Source: CAD feature listing. Evaluate the final solid. Frame: model axes, mm. A direction names the side the tool comes from. Round coordinates to 2 decimals unless told otherwise and drop trailing zeros. Order: outer loops, then holes, each group sorted by start corner. A loop starts at its lowest first (then second) coordinate and runs counter-clockwise, first axis right, second up. Notation, with made-up numbers: (54.25, 87) -> (68.25, 87) arc R27 ccw to (68.25, 104) -> close; hole circle Ø8 at (48.25, -36). An arc over 180 degrees is marked (long way). One line per item, written item: value. Start each with the question number.
1) Section A-A (y = 0). Return the cut outline in (x, z), and give its area (3 significant figures).
2) Pin query (flat end, axial travel): P1, Ø4, axis at x = 18, z = 536.5, coming from the -Y side; P2, Ø16, axis at y = 0, z = 325, coming from the -X side; P3, Ø15.5, axis at x = -24.5, y = 3, coming from the -Z side; P4, Ø6, axis at y = 0.5, z = 429.5, coming from the -X side. Return the tip coordinate at first contact, or that it passes through.
3) Section D-D (z = 522.5). Return the cut outline in (x, y), and give its area (3 significant figures).
4) Section B-B (x = 0). Return the cut outline in (y, z).
5) Ray query, L1, parallel to Z at x = -4, y = 0; L2, parallel to Z at x = -11, y = -9; L3, parallel to X at y = -5, z = 335. Return the intervals inside material, ascending.
6) Reachability of faces 5 (the face through (-4.336, -19.524, 524.865)), 6 (the face through (15, 0, 197)), 7 (the face through (0, -25, 197)), 8 (the face through (0, 25, 197)) from +Z, -Z, +X, -X, +Y, -Y: full face, straight path, thin tool, end or side. Return the list, or none.
7) Section C-C (z = 125). Return the cut outline in (x, y).
8) Mould query, pull axis Z, two halves, no side actions, for faces 1 (the face through (-22, 1, 400)), 2 (the face through (0.21, -1.302, 334.915)), 3 (the face through (-15, 0, 197)), 4 (the face through (0.21, -1.302, 34.915)). Classes: pulls with the +Z half, pulls with the -Z half, needs draft (parallel to the pull), parting line crosses it, or undercut.
```python
from build123d import *

# Parameters (mm, degrees)
ESQUISSE1_W             = 30
ESQUISSE1_H             = 50
BOSS_EXTRU_1_DEPTH      = 400
ESQUISSE2_R             = 29.154759474
BOSS_EXTRU_2_DEPTH      = 221
ESQUISSE3_R             = 20
ENL_V_MAT_EXTRU_1_DEPTH = 195
ENL_V_MAT_EXTRU_2_REACH = 625.25
ESQUISSE4_R             = 10


with BuildPart() as part:
    # Esquisse1 → Boss.-Extru.1 (new body)
    with BuildSketch(Plane.XY):
        Rectangle(ESQUISSE1_W, ESQUISSE1_H)
    extrude(amount=BOSS_EXTRU_1_DEPTH)

    # Esquisse2 → Boss.-Extru.2 (add)
    with BuildSketch(Plane.XY.offset(400)):
        with Locations(Location((0, 0, 0), (0, 0, 120.963756532))):
            Circle(ESQUISSE2_R)
    extrude(amount=BOSS_EXTRU_2_DEPTH)

    # Esquisse3 → Enlèv. mat.-Extru.1 (cut)
    with BuildSketch(Plane.XY.offset(621)):
        Circle(ESQUISSE3_R)
    extrude(amount=-ENL_V_MAT_EXTRU_1_DEPTH, mode=Mode.SUBTRACT)

    # Esquisse4 → Enlèv. mat.-Extru.2 (cut, up to next)
    with BuildSketch(Plane(origin=(15, 0, 0), x_dir=(0, 0, -1), z_dir=(1, 0, 0)), mode=Mode.PRIVATE) as enl_v_mat_extru_2_sk1:
        with Locations(Location((-25, 0, 0), (0, 0, 90))):
            Circle(ESQUISSE4_R)
    enl_v_mat_extru_2_tool1 = extrude(enl_v_mat_extru_2_sk1.sketch, amount=-ENL_V_MAT_EXTRU_2_REACH, mode=Mode.PRIVATE) & part.part
    # Esquisse4 → Enlèv. mat.-Extru.2 (cut, up to next)
    with BuildSketch(Plane(origin=(15, 0, 0), x_dir=(0, 0, -1), z_dir=(1, 0, 0)), mode=Mode.PRIVATE) as enl_v_mat_extru_2_sk2:
        with Locations(Location((-125, 0, 0), (0, 0, 90))):
            Circle(ESQUISSE4_R)
    enl_v_mat_extru_2_tool2 = extrude(enl_v_mat_extru_2_sk2.sketch, amount=-ENL_V_MAT_EXTRU_2_REACH, mode=Mode.PRIVATE) & part.part
    # Esquisse4 → Enlèv. mat.-Extru.2 (cut, up to next)
    with BuildSketch(Plane(origin=(15, 0, 0), x_dir=(0, 0, -1), z_dir=(1, 0, 0)), mode=Mode.PRIVATE) as enl_v_mat_extru_2_sk3:
        with Locations(Location((-325, 0, 0), (0, 0, 90))):
            Circle(ESQUISSE4_R)
    enl_v_mat_extru_2_tool3 = extrude(enl_v_mat_extru_2_sk3.sketch, amount=-ENL_V_MAT_EXTRU_2_REACH, mode=Mode.PRIVATE) & part.part
    add(enl_v_mat_extru_2_tool1.solids().sort_by_distance((15, 0, 25))[0], mode=Mode.SUBTRACT)
    add(enl_v_mat_extru_2_tool2.solids().sort_by_distance((15, 0, 125))[0], mode=Mode.SUBTRACT)
    add(enl_v_mat_extru_2_tool3.solids().sort_by_distance((15, 0, 325))[0], mode=Mode.SUBTRACT)


solid = part.part
```
Findings:
1. outline: (-29.15, 400) -> (-15, 400) -> (-15, 335) -> (15, 335) -> (15, 400) -> (29.15, 400) -> (29.15, 621) -> (20, 621) -> (20, 426) -> (-20, 426) -> (-20, 621) -> (-29.15, 621) -> close; (-15, 0) -> (15, 0) -> (15, 15) -> (-15, 15) -> close; (-15, 35) -> (15, 35) -> (15, 115) -> (-15, 115) -> close; (-15, 135) -> (15, 135) -> (15, 315) -> (-15, 315) -> close
1. area: 15,300 mm2
2. P1: y = -24.37
2. P2: through
2. P3: z = 400
2. P4: x = -29.15
3. outline: circle Ø58.31 at (0, 0); hole circle Ø40 at (0, 0)
3. area: 1,410 mm2
4. outline: (-29.15, 400) -> (-25, 400) -> (-25, 0) -> (25, 0) -> (25, 400) -> (29.15, 400) -> (29.15, 621) -> (20, 621) -> (20, 426) -> (-20, 426) -> (-20, 621) -> (-29.15, 621) -> close; hole circle Ø20 at (0, 25); hole circle Ø20 at (0, 125); hole circle Ø20 at (0, 325)
5. L1: 0 to 15, 35 to 115, 135 to 315, 335 to 426
5. L2: 0 to 20.64, 29.36 to 120.64, 129.36 to 320.64, 329.36 to 426
5. L3: -15 to 15
6. face 5: +Z
6. face 6: -Z, +X, +Y, -Y
6. face 7: -Z, +X, -X, -Y
6. face 8: -Z, +X, -X, +Y
7. outline: (-15, -25) -> (15, -25) -> (15, -10) -> (-15, -10) -> close; (-15, 10) -> (15, 10) -> (15, 25) -> (-15, 25) -> close
8. face 1: pulls with the -Z half
8. face 2: undercut
8. face 3: needs draft
8. face 4: undercut
